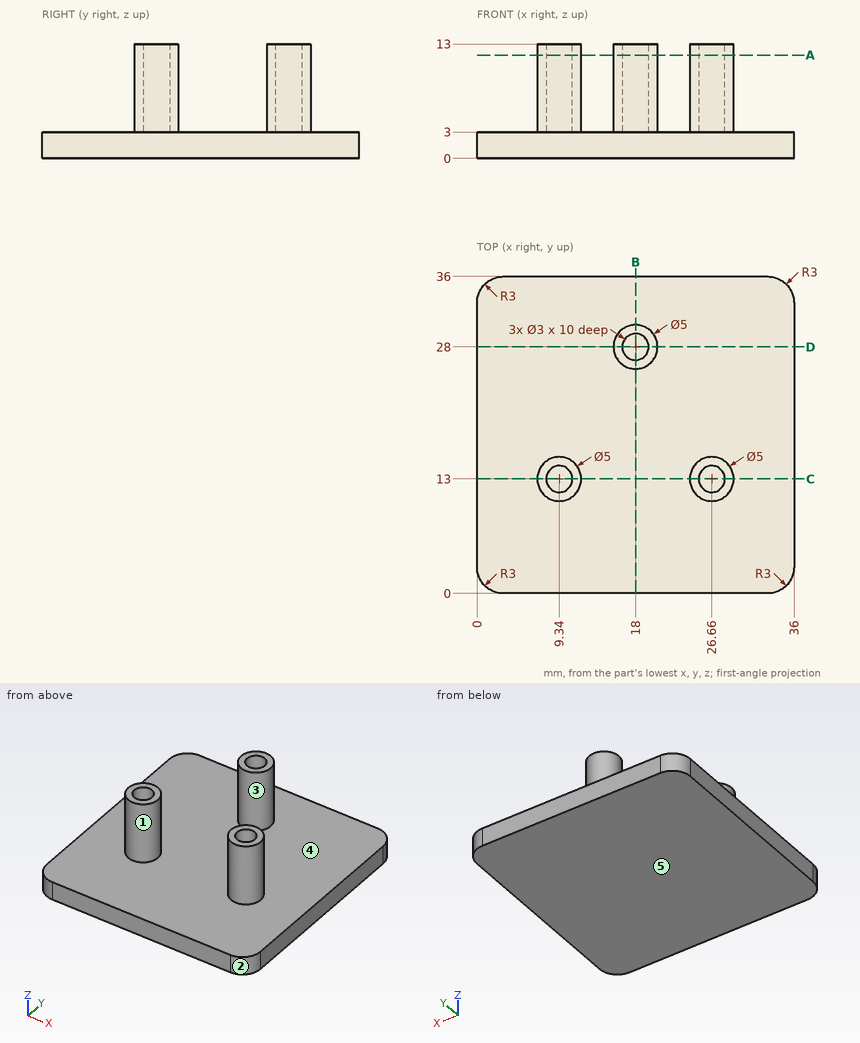
Can you work these out from the drawing? Everything is in mm from the part's minimum corner. A direction names the side the tool comes from. Coordinates: 2 decimals unless noted, no trailing zeros. Loops run counter-clockwise (first coordinate to the right, second up) from the corner with the lowest first, then second, coordinate; pieces in that order, holes last. Notation, with made-up numbers: M 55.5,-33 L 80.5,-33 A25 ccw 80.5,-20 Z; hole C 37,2 d6. An arc over 180 degrees is marked long. Put each result on its own line as item: value. Start each with the question number.
(1) Suppose I cut it at A-A on z = 11.75. Please give me the cut outline in (x, y), then the cut area to 3 significant figures.
(2) I need wall thicknesses on line 1 (Y direction, x = 9.5, z = 3.5) (1 decimal); line 2 (Y direction, x = 18, z = 8.25); line 3 (Z direction, x = 26.5, y = 6). Which ranges of each line are inside material? Lowest first, please. Write a range as from..to.
(3) Suppose I cut it at C-C on y = 13. Please give me the cut outline in (x, z).
(4) Thinking about a two-plate mould opening in X: for the marked faces 1, 2 and 3, which applies, pulls with the +X half, pulls with the -X half, needs draft (parallel to the pull), parting line crosses it, or undercut?
(5) Suppose I cut it at D-D on y = 28. Please give me the cut outline in (x, z), then the cut area to 3 significant figures.
(6) Suppose I cut it at B-B on x = 18. Please give me the cut outline in (y, z).
(7) For the marked faces 4 and 5, which set-ups out of +Z, -Z, +X, -X, +Y, -Y let a thin tool reach every point of the face, with its end or its side?
(8) Will these pins go through, and if not, where does the flat tip stop? P1, Ø4, axis at x = 15, z = 8, coming from the +Y side; P2, Ø3, axis at x = 8, z = 10.5, coming from the +Y side; P3, Ø6, axis at x = 19, z = 9, coming from the -Y side.
Solutions:
1. outline: C 9.34,13 d5; C 18,28 d5; C 26.66,13 d5; hole C 9.34,13 d3; hole C 18,28 d3; hole C 26.66,13 d3
1. area: 37.7 mm2
2. line 1: y = 10.5..11.5, 14.5..15.5
2. line 2: y = 25.5..26.5, 29.5..30.5
2. line 3: z = 0..3
3. outline: M 0,0 L 36,0 L 36,3 L 29.16,3 L 29.16,13 L 28.16,13 L 28.16,3 L 25.16,3 L 25.16,13 L 24.16,13 L 24.16,3 L 11.84,3 L 11.84,13 L 10.84,13 L 10.84,3 L 7.84,3 L 7.84,13 L 6.84,13 L 6.84,3 L 0,3 Z
4. face 1: undercut
4. face 2: pulls with the +X half
4. face 3: parting line crosses it
5. outline: M 0,0 L 36,0 L 36,3 L 20.5,3 L 20.5,13 L 19.5,13 L 19.5,3 L 16.5,3 L 16.5,13 L 15.5,13 L 15.5,3 L 0,3 Z
5. area: 128 mm2
6. outline: M 0,0 L 36,0 L 36,3 L 30.5,3 L 30.5,13 L 29.5,13 L 29.5,3 L 26.5,3 L 26.5,13 L 25.5,13 L 25.5,3 L 0,3 Z
7. face 4: +Z
7. face 5: -Z, +X, -X, +Y, -Y
8. P1: stops at y = 30.29
8. P2: stops at y = 15.5
8. P3: stops at y = 25.5
